from build123d import *

# Parameters (mm, degrees)
F2_R      = 2.5
F3_DEPTH  = 3
F4_W      = 3
F4_H      = 3
F4_W_2    = 41
F4_H_2    = 35
F5_DEPTH  = 114
F6_R      = 2.5
F7_DEPTH  = 3
F8_W      = 110
F8_H      = 20
F9_DEPTH  = 3
F10_W     = 47
F10_H     = 26
F10_W_2   = 48
F10_H_2   = 28
F11_DEPTH = 3
F13_DEPTH = 3
F14_SIZE  = 1
F16_W     = 48
F16_H     = 2
F16_W_2   = 47
F17_DEPTH = 1


with BuildPart() as f3:
    # F2 (on Right) → F3 (new body)
    with BuildSketch(Plane.YZ):
        with BuildLine():
            ThreePointArc((22.5, 35), (21.0355339059, 38.5355339059), (17.5, 40))
            Line((17.5, 40), (-19.5, 40))
            ThreePointArc((-19.5, 40), (-23.0355339059, 38.5355339059), (-24.5, 35))
            Line((-24.5, 35), (-24.5, -38))
            Line((-24.5, -38), (22.5, -38))
            Line((22.5, -38), (22.5, 35))
        make_face()
        with Locations((-12, 34.5)):
            Circle(F2_R, mode=Mode.SUBTRACT)
        with Locations((10, 34.5)):
            Circle(F2_R, mode=Mode.SUBTRACT)
    extrude(amount=F3_DEPTH)

    # F4 (on Right) → F5 (join)
    with BuildSketch(Plane.YZ):
        with Locations((21, -36.5)):
            Rectangle(F4_W, F4_H)
        with Locations((-1, -36.5)):
            Rectangle(F4_W_2, F4_H)
        with Locations((21, -17.5)):
            Rectangle(F4_W, F4_H_2)
        with Locations((-23, -36.5)):
            Rectangle(F4_W, F4_H)
        with Locations((-23, -17.5)):
            Rectangle(F4_W, F4_H_2)
    extrude(amount=-F5_DEPTH)

    # F6 (on face) → F7 (join)
    with BuildSketch(Plane(origin=(-114, 0, 0), x_dir=(0, -1, 0), z_dir=(-1, 0, 0))):
        with BuildLine():
            ThreePointArc((24.5, 35), (23.0355339059, 38.5355339059), (19.5, 40))
            Line((19.5, 40), (-17.5, 40))
            ThreePointArc((-17.5, 40), (-21.0355339059, 38.5355339059), (-22.5, 35))
            Line((-22.5, 35), (-22.5, -38))
            Line((-22.5, -38), (24.5, -38))
            Line((24.5, -38), (24.5, 35))
        make_face()
        with Locations((-10, 34.5)):
            Circle(F6_R, mode=Mode.SUBTRACT)
    extrude(amount=F7_DEPTH)

    # F8 (on face) → F9 (join)
    with BuildSketch(Plane.XZ.offset(24.5)):
        with Locations((-57, 10)):
            Rectangle(F8_W, F8_H)
    extrude(amount=-F9_DEPTH)

    # F10 (on face) → F11 (cut, through all)
    with BuildSketch(Plane.XZ.offset(24.5)):
        with Locations((-85.5, -19)):
            Rectangle(F10_W, F10_H)
        with Locations((-28.5, -19)):
            Rectangle(F10_W_2, F10_H_2)
    extrude(amount=-F11_DEPTH, mode=Mode.SUBTRACT)

    # F12 (on face) → F13 (cut, through all)
    with BuildSketch(Plane(origin=(0, 22.5, 0), x_dir=(-1, 0, 0), z_dir=(0, 1, 0))):
        with BuildLine():
            ThreePointArc((82, -26), (82.5857864376, -27.4142135624), (84, -28))
            Line((84, -28), (95, -28))
            ThreePointArc((95, -28), (96.4142135624, -27.4142135624), (97, -26))
            Line((97, -26), (97, -22))
            ThreePointArc((97, -22), (96.4142135624, -20.5857864376), (95, -20))
            Line((95, -20), (84, -20))
            ThreePointArc((84, -20), (82.5857864376, -20.5857864376), (82, -22))
            Line((82, -22), (82, -26))
        make_face()
        with BuildLine():
            ThreePointArc((17, -26), (17.5857864376, -27.4142135624), (19, -28))
            Line((19, -28), (30, -28))
            ThreePointArc((30, -28), (31.4142135624, -27.4142135624), (32, -26))
            Line((32, -26), (32, -22))
            ThreePointArc((32, -22), (31.4142135624, -20.5857864376), (30, -20))
            Line((30, -20), (19, -20))
            ThreePointArc((19, -20), (17.5857864376, -20.5857864376), (17, -22))
            Line((17, -22), (17, -26))
        make_face()
    extrude(amount=-F13_DEPTH, mode=Mode.SUBTRACT)

    # F14
    f14_edges = [f3.edges().sort_by_distance(p)[0] for p in [
        (-57, -24.5, -38),
        (3, -1, -38),
        (-57, 22.5, -38),
        (-117, -1, -38),
    ]]
    chamfer(f14_edges, length=F14_SIZE)

    # F16 (on face) → F17 (cut)
    with BuildSketch(Plane(origin=(0, -21.5, 0), x_dir=(-1, 0, 0), z_dir=(0, 1, 0))):
        with Locations((28.5, -34)):
            Rectangle(F16_W, F16_H)
        with Locations((85.5, -33)):
            Rectangle(F16_W_2, F16_H)
        with Locations((85.5, -5)):
            Rectangle(F16_W_2, F16_H)
        with Locations((28.5, -4)):
            Rectangle(F16_W, F16_H)
    extrude(amount=-F17_DEPTH, mode=Mode.SUBTRACT)


solid = f3.part
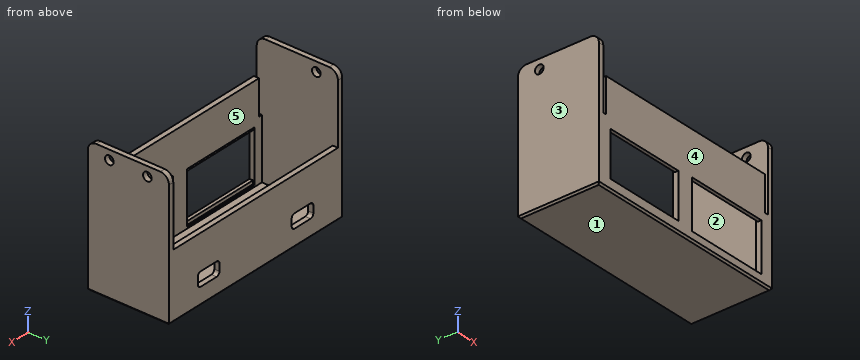
Source: CAD feature listing. Evaluate the final solid. Frame: model axes, mm. Face numbers are marked on the shaded views. A direction names the side the tool comes from. Give positions to 0.01 mm unless a question says otherwise; leave off trailing zeros. Write each loop counter-clockwise with the first axis right and the second up, starting at its lowest first coordinate (ties: lowest second). Pieces come first, ordered by that corner, then holes. Notation, with made-up numbers: M -0.5,54.5 L 6.5,54.5 A28 cw 6.5,92.5 Z; hole C 36,9.5 d4. An arc over 180 degrees is marked long. Answer as a JSON object with one key per item and string values.
Q1. Cut plane C-C, the plane x = -28. Return the cut outline in (y, z), then the cut area to 3 significant figures.
Geometry check:
{"outline": "M -24.5,-37 L -23.5,-38 L 21.5,-38 L 22.5,-37 L 22.5,-28 L 19.5,-28 L 19.5,-35 L -22.5,-35 L -22.5,-33 L -24.5,-33 Z; M -24.5,-5 L -22.5,-5 L -22.5,-3 L -21.5,-3 L -21.5,20 L -24.5,20 Z; M 19.5,-20 L 22.5,-20 L 22.5,0 L 19.5,0 Z", "area": "298 mm^2"}
Q2. Cut plane D-D, the plane z = -14. Return the cut outline in (x, y), then the cut area to 3 significant figures.
Geometry check:
{"outline": "M -117,-24.5 L -109,-24.5 L -109,-21.5 L -114,-21.5 L -114,19.5 L 0,19.5 L 0,-21.5 L -4.5,-21.5 L -4.5,-24.5 L 3,-24.5 L 3,22.5 L -117,22.5 Z; M -62,-24.5 L -52.5,-24.5 L -52.5,-21.5 L -62,-21.5 Z", "area": "681 mm^2"}
Q3. Mould query, pull axis X, two halves, no side actions, for the marked faces 3, 4 and 5. Classes: +X half, -X half, draft (parallel to the pull), parting line (faces both ways), or undercut.
Geometry check:
{"face 3": "-X half", "face 4": "draft", "face 5": "undercut"}
Q4. Access query for the marked faces 1 and 2. Directions: +Z, -Z, +X, -X, +Y, -Y. A direction counts if a zero-diameter tool reaches every point of the face in a straight line with its end or side. Return the directions, or none.
Geometry check:
{"face 1": "-Z, +X, -X, +Y, -Y", "face 2": "+Z"}
Q5. Cut plane A-A, the plane y = -12. Return the cut outline in (x, z).
Geometry check:
{"outline": "M -117,-37 L -116,-38 L 2,-38 L 3,-37 L 3,32 L 0,32 L 0,-35 L -114,-35 L -114,40 L -117,40 Z; M 0,37 L 3,37 L 3,40 L 0,40 Z"}
Q6. Contact query for flat-ended pins moving along their axis: P1, Ø8, axis at x = -58, y = -0.5, coming from the +Z side; P2, Ø0.9, axis at x = -51, y = 21, coming from the +Z side; P3, Ø2, axis at x = -87, y = -23, coming from the +Z side. Output: stop coordinate, or through.
Geometry check:
{"P1": "stops at z = -35", "P2": "stops at z = 0", "P3": "stops at z = 20"}
Q7. Ray query, line 1 along X through (y, z) = (15, 35); line 2 along Z through (x, y) = (1.45, -12); line 3 along Z through (x, y) = (-82, -14.5). Return the intervals inside material, ascending.
Geometry check:
{"line 1": "x = -117 to -114, 0 to 3", "line 2": "z = -38 to 32, 37 to 40", "line 3": "z = -38 to -35"}
Q8. Cut plane B-B, the plane z = 16.5. Return the cut outline in (x, y), then the cut area to 3 significant figures.
Geometry check:
{"outline": "M -117,-24.5 L -114,-24.5 L -114,22.5 L -117,22.5 Z; M -112,-24.5 L -2,-24.5 L -2,-21.5 L -112,-21.5 Z; M 0,-24.5 L 3,-24.5 L 3,22.5 L 0,22.5 Z", "area": "612 mm^2"}
